Build history of the part. All positions in model axes, mm. Round coordinates to 2 decimals unless told otherwise and drop trailing zeros. Write each loop counter-clockwise with the first axis right and the second up, starting at its lowest first coordinate (ties: lowest second). Pieces come first, ordered by that corner, then holes. Notation, with made-up numbers: (39, 22) -> (85, 22) arc R19 ccw to (85, 35) -> close; hole circle Ø7 at (43.5, -27.5). An arc over 180 degrees is marked (long way). One line per question, with ' | ' between items.
from build123d import *

# Parameters (mm, degrees)
SKETCH_1_R      = 448.7
EXTRUDE_2_DEPTH = 16


with BuildPart() as part:
    # Эскиз1 → Бобышка-Вытянуть2 (new body)
    with BuildSketch(Plane(origin=(0, 0, 0), x_dir=(1, 0, 0), z_dir=(0, 1, 0))):
        with BuildLine():
            Line((-344.32913914, 638.733962842), (-328.594635558, 635.831309398))
            Line((-328.594635558, 635.831309398), (-324.978198629, 655.435041258))
            ThreePointArc((-324.978198629, 655.435041258), (-19.068388145, 453.638466212), (60.542297577, 95.916774711))
            Line((60.542297577, 95.916774711), (40.882449344, 99.197669255))
            Line((40.882449344, 99.197669255), (37.979795899, 83.463165673))
            Line((37.979795899, 83.463165673), (57.516225139, 79.513249965))
            ThreePointArc((57.516225139, 79.513249965), (-144.23681545, -226.079457497), (-501.65610266, -305.720184329))
            Line((-501.65610266, -305.720184329), (-498.386954822, -286.060743027))
            Line((-498.386954822, -286.060743027), (-514.12229676, -283.162637766))
            Line((-514.12229676, -283.162637766), (-518.061372416, -302.703594153))
            ThreePointArc((-518.061372416, -302.703594153), (-823.9309706, -100.894655009), (-903.52528096, 256.803268902))
            Line((-903.52528096, 256.803268902), (-883.865432727, 253.522374358))
            Line((-883.865432727, 253.522374358), (-880.962779283, 269.256877941))
            Line((-880.962779283, 269.256877941), (-900.566511143, 272.873314869))
            ThreePointArc((-900.566511143, 272.873314869), (-698.769936097, 578.783125354), (-341.048244596, 658.393811076))
            Line((-341.048244596, 658.393811076), (-344.32913914, 638.733962842))
        make_face()
        with Locations((-421.491491692, 176.360021807)):
            Circle(SKETCH_1_R, mode=Mode.SUBTRACT)
    extrude(amount=EXTRUDE_2_DEPTH)


solid = part.part
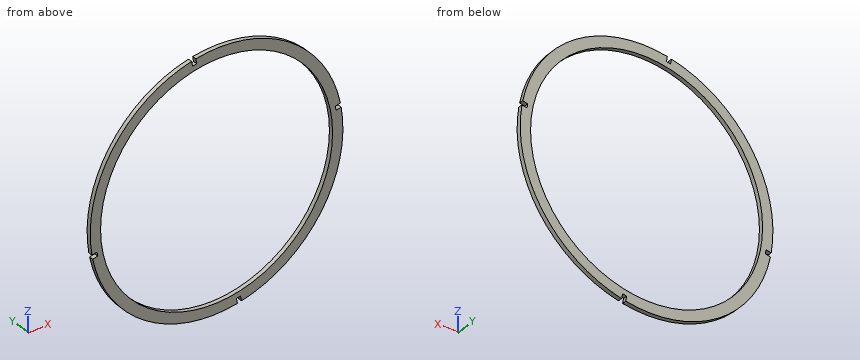
(1) Slice it at B-B (z = -436.5). Write the cut outline in (x, y), then the cut area to 3 significant figures.
Calculated:
outline: (-835.2, 0) -> (-787.09, 0) -> (-787.09, 16) -> (-835.2, 16) -> close; (-55.9, 0) -> (-7.78, 0) -> (-7.78, 16) -> (-55.9, 16) -> close | area: 1,540 mm2
(2) Wall check: line 1 (Z direction, x = -718.5, y = 3); line 2 (X direction, y = 4.75, z = -380); line 3 (X direction, y = 4, z = -122). Give the ranges that are in metal, low to high. Write a range as from..to.
Calculated:
line 1: -564.45..-512.69, 159.97..211.73 | line 2: -865.74..-821.32, -21.66..22.76 | line 3: -907.16..-866.89, 23.9..64.18
(3) Slice it at A-A (x = -664). Write the cut outline in (y, z).
Calculated:
outline: (0, -600.64) -> (16, -600.64) -> (16, -553.88) -> (0, -553.88) -> close; (0, 201.16) -> (16, 201.16) -> (16, 247.92) -> (0, 247.92) -> close
(4) Slice it at C-C (y = 7.75). Write the cut outline in (x, z), then the cut area to 3 significant figures.
Calculated:
outline: (-903.53, -256.8) -> (-883.87, -253.52) -> (-880.96, -269.26) -> (-900.57, -272.87) arc R488.7 ccw to (-341.05, -658.39) -> (-344.33, -638.73) -> (-328.59, -635.83) -> (-324.98, -655.44) arc R488.7 ccw to (60.54, -95.92) -> (40.88, -99.2) -> (37.98, -83.46) -> (57.52, -79.51) arc R488.7 ccw to (-501.66, 305.72) -> (-498.39, 286.06) -> (-514.12, 283.16) -> (-518.06, 302.7) arc R488.7 ccw to start; hole circle Ø897.4 at (-421.49, -176.36) | area: 116,000 mm2
(5) Drop flat-ended pins along their axis: pin 1 (1.5 mm diameter, centred on x = -292.5, y = 7.5, fed in from +Z); pin 2 (6 mm diameter, centred on x = -533, y = 13, fed in from -Z); pin 3 (1.5 mm diameter, centred on x = -565.5, y = 9.5, fed in from +Z). Give the stop position or say it passes through.
Calculated:
pin 1: z = 295.21 | pin 2: z = -652.86 | pin 3: z = 290.87
